The drawing under review shows one solid part. Ordinate dimensions are in mm from its lowest x, y, z. A direction names the side the tool comes from. Round coordinates to 2 decimals unless told otherwise and drop trailing zeros. Order: outer loops, then holes, each group sorted by start corner. A loop starts at its lowest first (then second) coordinate and runs counter-clockwise, first axis right, second up.
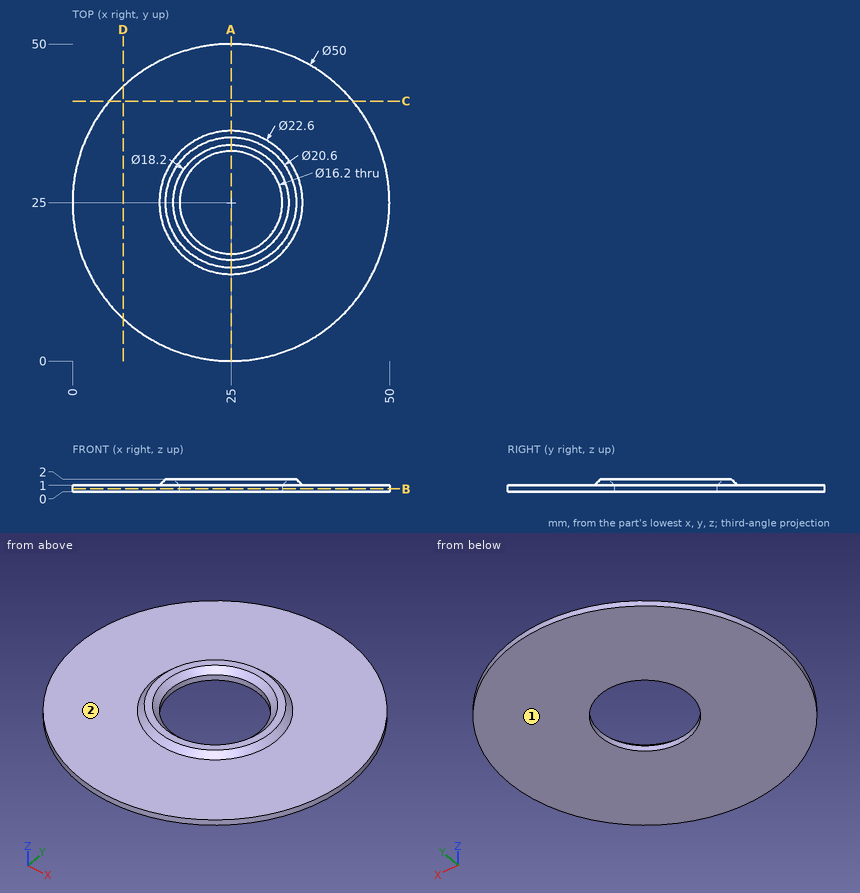
(1) We need section B-B (z = 0.45). Give the boundary of the cut face in (x, y), and give its area (3 significant figures).
(2) We need section A-A (x = 25). Give the boundary of the cut face in (y, z), and give its area (3 significant figures).
(3) Tool access review of the marked faces 1 and 2: name each direction out of +Z, -Z, +X, -X, +Y, -Y from which nothing blocks a thin tool from reaching the whole face with its end or side.
(4) To check wall thickness, follow L1, parallel to Y at x = 25, z = 0.75; L2, parallel to X at y = 20, z = 1.85; L3, parallel to Z at x = 36.5, y = 35. State the ranges of each line that lie inside material, in increasing order.
(5) Clearance check with flat-ended pins moving along their axes: P1, Ø6, axis at x = 24.5, y = 8.5, coming from the -Z side; P2, Ø3, axis at x = 38, y = 27.5, coming from the +Z side. State where each tip first meets the part, or that it passes through.
(6) We need section D-D (x = 8). Give the boundary of the cut face in (y, z).
(7) We need section C-C (y = 41). Give the boundary of the cut face in (x, z).
Verdict:
1. outline: circle Ø50 at (25, 25); hole circle Ø16.2 at (25, 25)
1. area: 1,760 mm2
2. outline: (0, 0) - (16.9, 0) - (16.9, 1) - (15.9, 2) - (14.7, 2) - (13.7, 1) - (0, 1) - close; (33.1, 0) - (50, 0) - (50, 1) - (36.3, 1) - (35.3, 2) - (34.1, 2) - (33.1, 1) - close
2. area: 38.2 mm2
3. face 1: -Z, +X, -X, +Y, -Y
3. face 2: +Z
4. L1: y = 0 to 16.9, 33.1 to 50
4. L2: x = 15.82 to 17.58, 32.42 to 34.18
4. L3: z = 0 to 1
5. P1: stops at z = 0
5. P2: stops at z = 1
6. outline: (6.67, 0) - (43.33, 0) - (43.33, 1) - (6.67, 1) - close
7. outline: (5.79, 0) - (44.21, 0) - (44.21, 1) - (5.79, 1) - close
